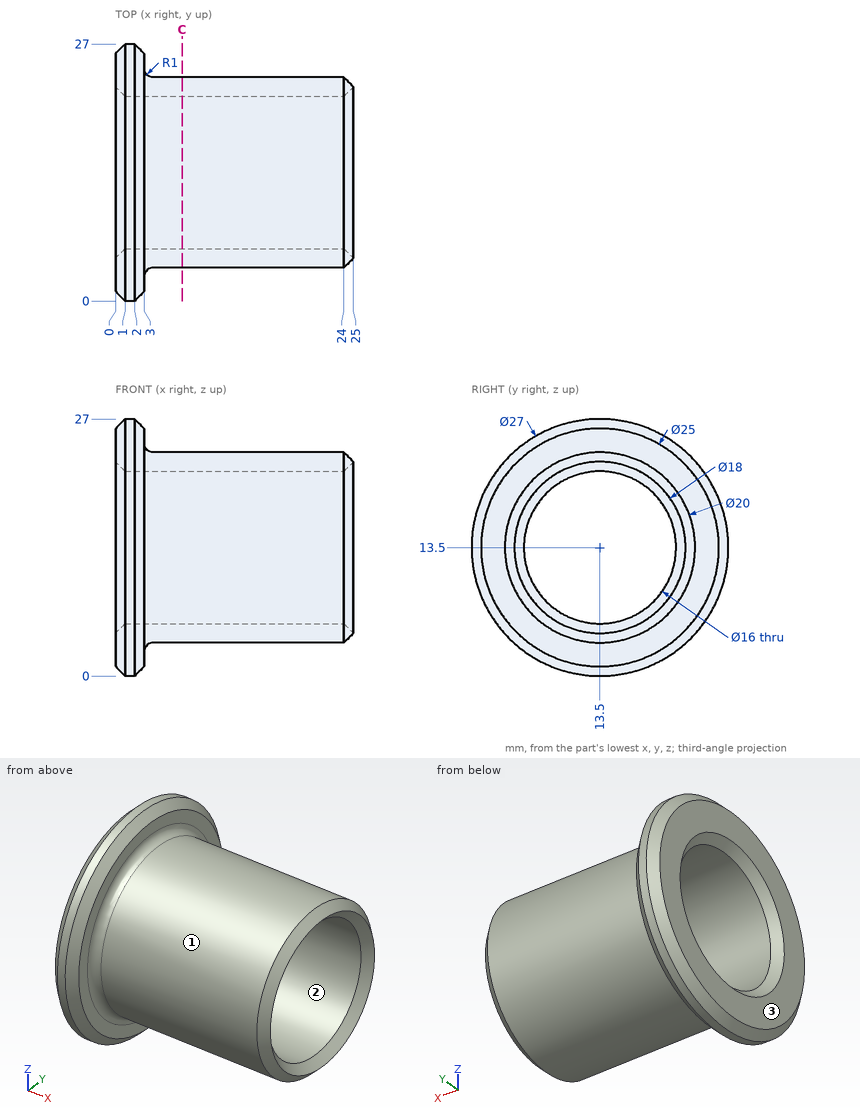
The drawing under review shows one solid part. Ordinate dimensions are in mm from its lowest x, y, z. Give positions to 0.01 mm unless a question says otherwise; leave off trailing zeros. Write each loop counter-clockwise with the first axis right and the second up, starting at its lowest first coordinate (ties: lowest second). Pieces come first, ordered by that corner, then holes. Notation, with made-up numbers: (-40, -17.75) -> (9, -17.75) arc R27 ccw to (9, 9.25) -> close; hole circle Ø6 at (79.25, 71.25). An arc over 180 degrees is marked (long way). Answer in a Markdown table with one row per item.
(1) Mouldability with a two-part tool opening along Y and no side actions: class the marked faces 1, 2 and 3 as +Y half, -Y half, draft (parallel to the pull), parting line (faces both ways), or undercut.
Results:
| item | result |
|---|---|
| face 1 | parting line |
| face 2 | undercut |
| face 3 | draft |
(2) Consider section C-C (x = 7). State the section outline as (y, z) points.
Results:
| item | result |
|---|---|
| outline | circle Ø20 at (13.5, 13.5); hole circle Ø16 at (13.5, 13.5) |
(3) Clearance check with flat-ended pins moving along their axes: pin 1 (10 mm diameter, centred on x = 16, y = 21, fed in from +Z); pin 2 (7.5 mm diameter, centred on y = 11, z = 17.5, fed in from +X); pin 3 (2 mm diameter, centred on x = 7.5, z = 3.5, fed in from -Y). State where each tip first meets the part, or that it passes through.
Results:
| item | result |
|---|---|
| pin 1 | z = 23.18 |
| pin 2 | x = 24.47 |
| pin 3 | y = 9.14 |
(4) To check wall thickness, follow probe 1 along Y at (x, z) = (18.25, 13.5); probe 2 along X at (y, z) = (3, 9); probe 3 along Y at (x, z) = (2.5, 6.25). State the ranges of each line that lie inside material, in increasing order.
Results:
| item | result |
|---|---|
| probe 1 | 3.5 to 5.5, 21.5 to 23.5 |
| probe 2 | 0 to 3 |
| probe 3 | 2.71 to 10.12, 16.88 to 24.29 |
